from build123d import *

# Parameters (mm, degrees)
F0_R     = 38.1
F1_DEPTH = 12.7
F2_R     = 19.05
F3_DEPTH = 38.1
F4_R     = 10.474618
F5_DEPTH = 12.7
F6_R     = 5.428581
F6_R_2   = 5.923411
F6_R_3   = 5.637256
F6_R_4   = 5.703751
F7_DEPTH = 12.701
F8_R     = 5.809223
F9_DEPTH = 63.501


with BuildPart() as f1:
    # F0 (on Top) → F1 (new body)
    with BuildSketch(Plane.XY):
        Circle(F0_R)
    extrude(amount=-F1_DEPTH)

    # F2 (on face) → F3 (join)
    with BuildSketch(Plane.XY):
        Circle(F2_R)
    extrude(amount=F3_DEPTH)

    # F4 (on face) → F5 (join)
    with BuildSketch(Plane.XY.offset(38.1)):
        Circle(F4_R)
    extrude(amount=F5_DEPTH)

    # F6 (on face) → F7 (cut, through all)
    with BuildSketch(Plane.XY):
        with Locations((0, -27.94018)):
            Circle(F6_R)
        with Locations((28.614422, 0)):
            Circle(F6_R_2)
        with Locations((0, 30.194912)):
            Circle(F6_R_3)
        with Locations((-30.750221, 0)):
            Circle(F6_R_4)
    extrude(amount=-F7_DEPTH, mode=Mode.SUBTRACT)

    # F8 (on face) → F9 (cut, through all)
    with BuildSketch(Plane.XY.offset(50.8)):
        Circle(F8_R)
    extrude(amount=-F9_DEPTH, mode=Mode.SUBTRACT)


solid = f1.part
Geometry check sheet. Reference: the model listing, model coordinates, mm. A direction names the side the tool comes from. Round coordinates to 2 decimals unless told otherwise and drop trailing zeros. Order: outer loops, then holes, each group sorted by start corner. A loop starts at its lowest first (then second) coordinate and runs counter-clockwise, first axis right, second up. Notation, with made-up numbers: M -23,67.25 L 19,67.25 A25 cw 19,81.25 Z; hole C 74,66 d4. An arc over 180 degrees is marked long. Answer in a Markdown table with one row per item.
(1) Go/stop test with flat-tipped pins: P1, Ø1.5, axis at y = 10.5, z = 14, coming from the -X side; P2, Ø12, axis at x = -26, y = 3.5, coming from the +Z side; P3, Ø1.5, axis at x = -18, z = -2, coming from the +Y side. Record where each tip stops, or that it passes through.
Responses:
| item | result |
|---|---|
| P1 | stops at x = -16.37 |
| P2 | stops at z = 0 |
| P3 | stops at y = 33.97 |
(2) Sectioned sample at A-A, the plane x = 0. Record the cut outline in (y, z), and give its area (3 significant figures).
Responses:
| item | result |
|---|---|
| outline | M -38.1,-12.7 L -33.37,-12.7 L -33.37,0 L -38.1,0 Z; M -22.51,-12.7 L -5.81,-12.7 L -5.81,50.8 L -10.47,50.8 L -10.47,38.1 L -19.05,38.1 L -19.05,0 L -22.51,0 Z; M 5.81,-12.7 L 24.56,-12.7 L 24.56,0 L 19.05,0 L 19.05,38.1 L 10.47,38.1 L 10.47,50.8 L 5.81,50.8 Z; M 35.83,-12.7 L 38.1,-12.7 L 38.1,0 L 35.83,0 Z |
| area | 1,670 mm² |
(3) Sectioned sample at D-D, the plane z = 47.5. Record the cut outline in (x, y).
Responses:
| item | result |
|---|---|
| outline | C 0,0 d20.95; hole C 0,0 d11.62 |
(4) Draft check along X on faces 3 (the face through (8, -8, 38.1)), 4 (the face through (9.99, 3.15, 44.36)), 5 (the face through (-1.18, -33.24, -6.26)), 6 (the face through (-1.22, 24.69, -6.26)). Enter one of: released by +X, released by -X, zero draft, split by the parting line, or undercut.
Responses:
| item | result |
|---|---|
| face 3 | zero draft |
| face 4 | split by the parting line |
| face 5 | undercut |
| face 6 | undercut |
(5) Tool access check on faces 1 (the face through (7.9, 17.5, 0)), 2 (the face through (5, -5, 50.8)). Record the directions out of +Z, -Z, +X, -X, +Y, -Y that give a thin tool (end or side, any length) a straight path to the whole face; none if there is none.
Responses:
| item | result |
|---|---|
| face 1 | +Z |
| face 2 | +Z, +X, -X, +Y, -Y |
(6) Scan lines: probe 1 along Y at (x, z) = (0, -9.5); probe 2 along Y at (x, z) = (0, 37); probe 3 along Z at (x, y) = (29, 19.5). Record each from-to range of solid material in increasing order. Write a range as from..to.
Responses:
| item | result |
|---|---|
| probe 1 | y = -38.1..-33.37, -22.51..-5.81, 5.81..24.56, 35.83..38.1 |
| probe 2 | y = -19.05..-5.81, 5.81..19.05 |
| probe 3 | z = -12.7..0 |
(7) Sectioned sample at C-C, the plane y = 0. Record the cut outline in (x, z), and give its area (3 significant figures).
Responses:
| item | result |
|---|---|
| outline | M -38.1,-12.7 L -36.45,-12.7 L -36.45,0 L -38.1,0 Z; M -25.05,-12.7 L -5.81,-12.7 L -5.81,50.8 L -10.47,50.8 L -10.47,38.1 L -19.05,38.1 L -19.05,0 L -25.05,0 Z; M 5.81,-12.7 L 22.69,-12.7 L 22.69,0 L 19.05,0 L 19.05,38.1 L 10.47,38.1 L 10.47,50.8 L 5.81,50.8 Z; M 34.54,-12.7 L 38.1,-12.7 L 38.1,0 L 34.54,0 Z |
| area | 1,650 mm² |
(8) Sectioned sample at B-B, the plane y = -29.5. Record the cut outline in (x, z).
Responses:
| item | result |
|---|---|
| outline | M -24.11,-12.7 L -5.2,-12.7 L -5.2,0 L -24.11,0 Z; M 5.2,-12.7 L 24.11,-12.7 L 24.11,0 L 5.2,0 Z |
